from build123d import *
from build123d import SkipClean  # not in build123d's __all__

# Parameters (mm, degrees)
F1_DEPTH = 21
F2_R     = 8
F3_DEPTH = 1


with BuildPart() as f1:
    # F0 (on Front) → F1 (new body)
    with BuildSketch(Plane.XZ):
        with BuildLine():
            Line((-3.928567067, -0.6374265649), (-3.9488843202, -0.6374265649))
            ThreePointArc((-3.9488843202, -0.6374265649), (3.9997163197, 0.0476378244), (-3.9629458697, 0.5431942877))
            Line((-3.9629458697, 0.5431942877), (-3.928567067, 0.5431942877))
            ThreePointArc((-3.928567067, 0.5431942877), (1.0007401595, -0.0471161386), (-3.928567067, -0.6374265649))
        make_face()
    extrude(amount=F1_DEPTH)

    # F2 (on face) → F3 (join)
    with BuildSketch(Plane(origin=(0, 0, 0), x_dir=(-1, 0, 0), z_dir=(0, 1, 0))):
        Circle(F2_R)
        with BuildLine():
            ThreePointArc((3.928567067, 0.5431942877), (3.9815237333, 0.250147998), (3.9992598405, -0.0471161386))
            ThreePointArc((3.9992598405, -0.0471161386), (3.9815237333, -0.3443802752), (3.928567067, -0.6374265649))
            Line((3.928567067, -0.6374265649), (3.9488843202, -0.6374265649))
            ThreePointArc((3.9488843202, -0.6374265649), (-3.9997163197, 0.0476378244), (3.9629458697, 0.5431942877))
            Line((3.9629458697, 0.5431942877), (3.928567067, 0.5431942877))
        make_face(mode=Mode.SUBTRACT)
    with SkipClean():  # cleaning this boolean's faces spoils the solid; the shape is the same uncleaned
        extrude(amount=-F3_DEPTH)


solid = f1.part
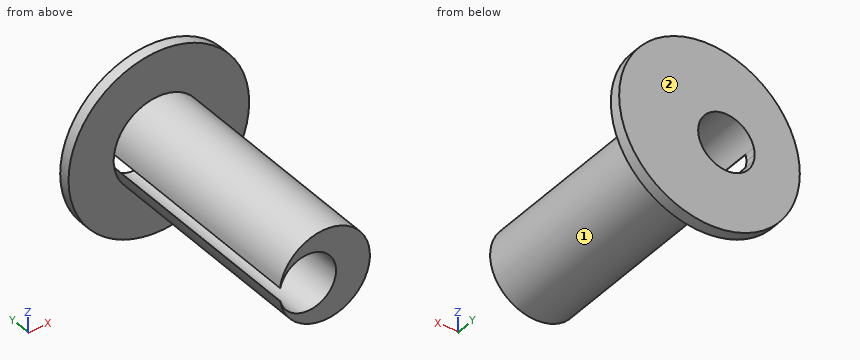
Source: CAD feature listing. Evaluate the final solid. Frame: model axes, mm. Face numbers are marked on the shaded views. A direction names the side the tool comes from. Round coordinates to 2 decimals unless told otherwise and drop trailing zeros. Loops run counter-clockwise (first coordinate to the right, second up) from the corner with the lowest first, then second, coordinate; pieces in that order, holes last.
Q1. Section B-B, the plane z = -1. Return loops of the section in (x, y).
Q2. Ray query, line 1 (Z direction, x = -2.75, y = -13.5); line 2 (Y direction, x = -3.5, z = 3.25); line 3 (Z direction, x = -2, y = -16.75). Return the intervals inside material, ascending.
Q3. Section A-A, the plane x = 0. Return loops of the section in (y, z).
Q4. Section C-C, the plane z = -3.5. Return loops of the section in (x, y).
Q5. First-contact query: P1, Ø6, axis at x = 6.5, y = -11.5, coming from the +Z side; P2, Ø4, axis at x = 3.5, y = -13, coming from the +Z side; P3, Ø6, axis at y = -3.5, z = 3, coming from the +X side. Flat tips, straight axial feed; report the tip coordinate or a pass-through.
Q6. Access query for the marked faces 1 and 2. Directions: +Z, -Z, +X, -X, +Y, -Y. A direction counts if a zero-diameter tool reaches every point of the face in a straight line with its end or side. Return the directions, or none.
Solutions:
1. outline: (-7.94, -1) - (-3.87, -1) - (-3.87, -21) - (-3.81, -21) - (-3.81, 0) - (-7.94, 0) - close; (0.81, -21) - (3.87, -21) - (3.87, -1) - (7.94, -1) - (7.94, 0) - (0.81, 0) - close
2. line 1: z = -2.9 to -2.21, 2.12 to 2.9
2. line 2: y = -1 to 0
2. line 3: z = -3.46 to -2.5, 2.4 to 3.46
3. outline: (-21, -4) - (-1, -4) - (-1, -8) - (0, -8) - (0, -2.05) - (-21, -2.05) - close; (-21, 1.95) - (0, 1.95) - (0, 8) - (-1, 8) - (-1, 4) - (-21, 4) - close
4. outline: (-7.19, -1) - (-1.94, -1) - (-1.94, -21) - (1.94, -21) - (1.94, -1) - (7.19, -1) - (7.19, 0) - (-7.19, 0) - close
5. P1: stops at z = 1.94
5. P2: stops at z = 3.71
5. P3: stops at x = 7.89
6. face 1: -Y
6. face 2: +Z, -Z, +X, -X, +Y
